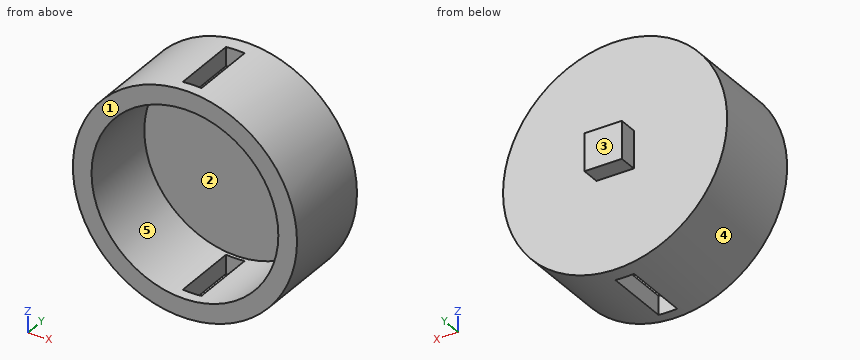
from build123d import *

# Parameters (mm, degrees)
SKETCH003_W  = 5
SKETCH003_H  = 18
PAD002_DEPTH = 37.5
SKETCH_R     = 30
PAD_DEPTH    = 12.5
SKETCH001_R  = 25
POCKET_DEPTH = 22
SKETCH002_W  = 10
SKETCH002_H  = 10
PAD001_DEPTH = 5


with BuildPart() as pad002:
    # Sketch003 → Pad002 (new body, symmetric)
    with BuildSketch(Plane.XY):
        with Locations((0, -0.5)):
            Rectangle(SKETCH003_W, SKETCH003_H)
    extrude(amount=PAD002_DEPTH, both=True)


with BuildPart() as cut:
    # Sketch → Pad (new body, symmetric)
    with BuildSketch(Plane.XZ):
        Circle(SKETCH_R)
    extrude(amount=PAD_DEPTH, both=True)

    # Sketch001 → Pocket (cut)
    with BuildSketch(Plane.XZ.offset(12.5)):
        Circle(SKETCH001_R)
    extrude(amount=-POCKET_DEPTH, mode=Mode.SUBTRACT)

    # Sketch002 → Pad001 (new body)
    with BuildSketch(Plane(origin=(0, 12.5, 0), x_dir=(1, 0, 0), z_dir=(0, 1, 0))):
        Rectangle(SKETCH002_W, SKETCH002_H)
    extrude(amount=PAD001_DEPTH)

    # Cut: cut Pad002
    add(pad002.part, mode=Mode.SUBTRACT)


solid = cut.part
Model file for the job. Use its own axes, mm. Face numbers are marked on the shaded views. A direction names the side the tool comes from. Round coordinates to 2 decimals unless told otherwise and drop trailing zeros. Loops run counter-clockwise (first coordinate to the right, second up) from the corner with the lowest first, then second, coordinate; pieces in that order, holes last. Notation, with made-up numbers: M -37,42 L -12,42 A34 ccw -12,74 Z; hole C -29.5,87 d8. An arc over 180 degrees is marked long. One line per question, with ' | ' between items.
1) Mould opens along Z. For the marked faces 3, 4 and 5 say: +Z half, -Z half, draft (parallel to the pull), parting line (faces both ways), or undercut.
Solved:
face 3: draft | face 4: parting line | face 5: undercut
2) Band-saw the part on D-D (x = 24). Give the cut face in (y, z).
Solved:
outline: M -12.5,-18 L 12.5,-18 L 12.5,18 L -12.5,18 L -12.5,7 L 9.5,7 L 9.5,-7 L -12.5,-7 Z
3) 3-axis set-ups, long thin cutter, end or side, ignore diameter. For the marked faces 1 and 2: which of +Z, -Z, +X, -X, +Y, -Y reach the whole face in a straight line?
Solved:
face 1: +Z, -Z, +X, -X, -Y | face 2: -Y
4) Band-saw the part on C-C (z = 0). Give the cut face in (x, y).
Solved:
outline: M -30,-12.5 L -25,-12.5 L -25,9.5 L 25,9.5 L 25,-12.5 L 30,-12.5 L 30,12.5 L 5,12.5 L 5,17.5 L -5,17.5 L -5,12.5 L -30,12.5 Z
5) Flat gauge pins, fed straight in: pin 1 (2 mm diameter, centred on x = -16.5, y = 6, fed in from -Z); pin 2 (2.5 mm diameter, centred on y = 15, z = -0.5, fed in from +X); pin 3 (5 mm diameter, centred on x = 0, z = -2, fed in from -Y). Where does each tip first touch, or does it go through?
Solved:
pin 1: stops at z = -25.69 | pin 2: stops at x = 5 | pin 3: stops at y = 9.5
6) Band-saw the part on B-B (x = 0). Give the cut face in (y, z), then the cut area to 3 significant figures.
Solved:
outline: M -12.5,-30 L -9.5,-30 L -9.5,-25 L -12.5,-25 Z; M -12.5,25 L -9.5,25 L -9.5,30 L -12.5,30 Z; M 8.5,-30 L 12.5,-30 L 12.5,-5 L 17.5,-5 L 17.5,5 L 12.5,5 L 12.5,30 L 8.5,30 L 8.5,25 L 9.5,25 L 9.5,-25 L 8.5,-25 Z | area: 270 mm²
7) Drill centre lines: line 1 along Y through (x, z) = (4, -12.5); line 2 along Z through (x, y) = (7, 7.25); line 3 along Z through (x, y) = (-9, -2.5). Where is each one in solid material? Low to high.
Solved:
line 1: y = 9.5 to 12.5 | line 2: z = -29.17 to -24, 24 to 29.17 | line 3: z = -28.62 to -23.32, 23.32 to 28.62
